Here's how the part is built. I have some questions about the finished solid (model axes, mm). A direction names the side the tool comes from. Round coordinates to 2 decimals unless told otherwise and drop trailing zeros. Write each loop counter-clockwise with the first axis right and the second up, starting at its lowest first coordinate (ties: lowest second). Pieces come first, ordered by that corner, then holes. Notation, with made-up numbers: (-22, 72.5) - (-14, 72.5) arc R4 cw to (-14, 77.5) - close; hole circle Ø7 at (88.5, -30). An arc over 180 degrees is marked (long way). Use one line per item in the form item = value. Start each with the question number.
1. I want a section at A-A, the plane z = 1.75. List the corners of the cut face in (x, y) for me, plus the area to 3 significant figures.
2. Which directions (+Z, -Z, +X, -X, +Y, -Y) give clear straight access to the entire face, cutting with the end or side of a thin tool? Please do faces 5 (the flat face through (-50, 7.5, 5)), 6 (the flat face through (-29, -7, 11)), 7 (the flat face through (-35, -6.3, 4)), 8 (the flat face through (-20.656, 7, 7)).
3. If I drill on line 1 along Y through (x, z) = (-36, 4); line 2 along X through (y, z) = (5.5, 6.5); line 3 along X through (y, z) = (1.25, 0.75), over which ranges is the centre line in solid material (lowest first)?
4. We'd pull the mould along Z, two halves only. Please class faces 1 (the flat face through (-38.6, 9.5, 8)), 2 (the flat face through (-29, -7, 5)), 3 (the flat face through (-44, -7, 2.5)), 4 (the flat face through (-29.062, 9, 4)): +Z half, -Z half, draft (parallel to the pull), parting line (faces both ways), or undercut.
5. Will these pins go through, and if not, where does the flat tip stop? pin 1 (0.6 mm diameter, centred on y = -7, z = 7.5, fed in from -X); pin 2 (0.6 mm diameter, centred on x = -43.5, y = 7, fed in from +Z); pin 3 (8 mm diameter, centred on x = -37, y = 0, fed in from -Z); pin 4 (6.5 mm diameter, centred on y = 11, z = 5, fed in from -X).
6. I want a section at D-D, the plane z = 7.5. State how many separate pieces and enclosed holes the cut face has, plus the area to 3 significant figures.
7. I want a section at C-C, the plane y = -1.75. List the corners of the cut face in (x, z) for me.
8. I want a section at B-B, the plane x = -40. List the corners of the cut face in (y, z) for me, plus the area to 3 significant figures.
```python
from build123d import *

# Parameters (mm, degrees)
F0_W      = 38
F0_H      = 15
F1_DEPTH  = 15
F2_T      = -1.2
F3_W      = 13
F3_H      = 6
F3_W_2    = 6
F3_H_2    = 8.5
F4_DEPTH  = 1.2
F5_DEPTH  = 1.2
F6_DEPTH  = 25
F7_R      = 4
F8_W      = 28
F8_H      = 13.8
F9_DEPTH  = 1.2
F10_W     = 10
F10_H     = 10
F11_DEPTH = 8
F12_T     = -0.8
F13_DEPTH = 25
F14_W     = 9.5933079185
F14_H     = 1.2
F15_DEPTH = 1.2


with BuildPart() as f1:
    # F0 (on Top) → F1 (new body)
    with BuildSketch(Plane.XY):
        with Locations((-34.6555788131, 0)):
            Rectangle(F0_W, F0_H)
    extrude(amount=F1_DEPTH)

    # F2 (hollow: no face is removed)
    offset(amount=F2_T, mode=Mode.SUBTRACT)

    # F3 (on face) → F4 (cut, through all)
    with BuildSketch(Plane.XZ.offset(7.5)):
        with Locations((-29.1555788131, 8)):
            Rectangle(F3_W, F3_H)
        with Locations((-43.6555788131, 6.75)):
            Rectangle(F3_W_2, F3_H_2)
    extrude(amount=-F4_DEPTH, mode=Mode.SUBTRACT)

    # F5 (cut, through all): a face of the model
    f5_faces = [f1.faces().sort_by_distance(p)[0] for p in [
        (-34.6555788131, 0, 15),
    ]]
    extrude(f5_faces, amount=-F5_DEPTH, mode=Mode.SUBTRACT)

    # F6 (cut): a face of the model
    f6_faces = [f1.faces().sort_by_distance(p)[0] for p in [
        (-34.6555788131, 0, 1.2),
    ]]
    extrude(f6_faces, amount=-F6_DEPTH, mode=Mode.SUBTRACT)

    # F7
    f7_edges = [f1.edges().sort_by_distance(p)[0] for p in [
        (-15.655579, -7.5, 6.9),
        (-52.455579, -6.3, 6.9),
        (-53.655579, -7.5, 6.9),
        (-16.855579, -6.3, 6.9),
    ]]
    fillet(f7_edges, radius=F7_R)

    # F8 (on face) → F9 (cut, through all)
    with BuildSketch(Plane(origin=(0, 7.5, 0), x_dir=(-1, 0, 0), z_dir=(0, 1, 0))):
        with Locations((34.6555788131, 6.9)):
            Rectangle(F8_W, F8_H)
    extrude(amount=-F9_DEPTH, mode=Mode.SUBTRACT)



with BuildPart() as f11:
    # F10 (on Top) → F11 (new body)
    with BuildSketch(Plane.XY):
        with Locations((-34.0622708946, 9.4726205524)):
            Rectangle(F10_W, F10_H)
    extrude(amount=F11_DEPTH)

    # F12
    f12_openings = [f11.faces().sort_by_distance(p)[0] for p in [
        (-34.062271, 9.472621, 0),
    ]]
    offset(amount=F12_T, openings=f12_openings)

    # F13 (cut): a face of the model
    f13_faces = [f11.faces().sort_by_distance(p)[0] for p in [
        (-34.0622708946, 9.4726205524, 7.2),
    ]]
    extrude(f13_faces, amount=-F13_DEPTH, mode=Mode.SUBTRACT)


with BuildPart() as f1_1:
    add(f1.part)

    add(f11.part)  # F15 merges F11
    # F14 (on Top) → F15 (join)
    with BuildSketch(Plane.XY):
        with Locations((-43.8589248539, 6.9)):
            Rectangle(F14_W, F14_H)
    extrude(amount=F15_DEPTH)


solid = f1_1.part
```
Model answer:
q1.outline = (-53.66, -3.5) arc R4 ccw to (-49.66, -7.5) - (-19.66, -7.5) arc R4 ccw to (-15.66, -3.5) - (-15.66, 7.5) - (-20.66, 7.5) - (-20.66, 6.3) - (-16.86, 6.3) - (-16.86, -2.3) arc R4 cw to (-20.86, -6.3) - (-48.46, -6.3) arc R4 cw to (-52.46, -2.3) - (-52.46, 6.3) - (-48.66, 6.3) - (-48.66, 7.5) - (-53.66, 7.5) - close; (-39.06, 4.47) - (-29.06, 4.47) - (-29.06, 14.47) - (-39.06, 14.47) - close; hole (-38.26, 5.27) - (-29.86, 5.27) - (-29.86, 13.67) - (-38.26, 13.67) - close
q1.area = 117 mm2
q2.face_5 = +Z, -Z, -X, +Y
q2.face_6 = +Y, -Y
q2.face_7 = +Z, -Z
q2.face_8 = +Z, -Z, +Y
q3.line_1 = -7.5 to -6.3, 4.47 to 5.27, 13.67 to 14.47
q3.line_2 = -53.66 to -52.46, -39.06 to -38.26, -29.86 to -29.06, -16.86 to -15.66
q3.line_3 = -53.66 to -52.46, -16.86 to -15.66
q4.face_1 = +Z half
q4.face_2 = undercut
q4.face_3 = undercut
q4.face_4 = draft
q5.pin_1 = -52.06
q5.pin_2 = 1.2
q5.pin_3 = through
q5.pin_4 = -39.06
q6.separate_pieces = 4
q6.enclosed_holes = 1
q6.area = 94.5 mm2
q7.outline = (-53.66, 0) - (-52.46, 0) - (-52.46, 13.8) - (-53.66, 13.8) - close; (-16.86, 0) - (-15.66, 0) - (-15.66, 13.8) - (-16.86, 13.8) - close
q8.outline = (-7.5, 0) - (-6.3, 0) - (-6.3, 13.8) - (-7.5, 13.8) - close; (6.3, 0) - (7.5, 0) - (7.5, 1.2) - (6.3, 1.2) - close
q8.area = 18.0 mm2
